The model under review builds one solid part; all positions refer to its coordinate system, in mm. A direction names the side the tool comes from. Round coordinates to 2 decimals unless told otherwise and drop trailing zeros. Order: outer loops, then holes, each group sorted by start corner. A loop starts at its lowest first (then second) coordinate and runs counter-clockwise, first axis right, second up. Notation, with made-up numbers: M 38.25,42.5 L 52.25,42.5 A23 ccw 52.25,60.5 Z; hole C 36.25,65 d10. An arc over 180 degrees is marked long. Use a Markdown table: item, result. Add a question column.
1. Consider section B-B on x = 17. State the section outline as (y, z) points, then the cut area to 3 significant figures.
2. To check wall thickness, follow probe 1 along X at (y, z) = (-95.95, -66); probe 2 along Y at (x, z) = (22, -7); probe 3 along Z at (x, y) = (-8.5, -88). State the ranges of each line that lie inside material, in increasing order.
3. Consider section C-C on z = -43. State the section outline as (x, y) points, then the cut area to 4 significant figures.
4. Consider section D-D on y = -75.5. State the section outline as (x, z) points, then the cut area to 4 significant figures.
5. The part is to be moulded in two halves that separate along X. For faces 6 (the flat face through (15, -96, -70)), 7 (the flat face through (-15.079, -94, -35)), 8 (the flat face through (-3.079, -84, 1)), 9 (the flat face through (38.421, -83, 1)), say which applies: +X half, -X half, draft (parallel to the pull), parting line (faces both ways), or undercut.
6. Insertion check: P1, Ø1.5, axis at x = 19, y = -103, coming from the -Z side; P2, Ø1.7, axis at x = -21.08, y = -115.76, coming from the -Z side; P3, Ø7, axis at y = -92.5, z = -46.5, coming from the -X side; P4, Ø6, axis at x = 6, z = -29, coming from the +Y side. Each pin has a flat end and moves straight along its axis. Give the tip position at first contact, or say it passes through.
7. Consider section A-A on z = -66. State the section outline as (x, y) points.
8. For faces 1 (the flat face through (14, -118.756, 1)), 2 (the flat face through (-13.079, -92, -35)), 3 (the flat face through (27, -76.756, 1)), 4 (the flat face through (53.421, -81, 1)), 5 (the flat face through (44.421, -94, -35)), list the 3-axis set-ups (+Z, -Z, +X, -X, +Y, -Y) from which the entire face can be reached by the end or side of a thin tool; tool diameter is ignored.
from build123d import *

# Parameters (mm, degrees)
SZKIC1_W                    = 77.5
SZKIC1_H                    = 77
SZKIC1_W_2                  = 13.5
SZKIC1_H_2                  = 11
DODANIE_WYCI_GNI_CIE1_DEPTH = 3
DODANIE_WYCI_GNI_CIE3_DEPTH = 70
SZKIC2_R                    = 1.4
WYTNIJ_WYCI_GNI_CIE1_DEPTH  = 3
SZKIC4_R                    = 1.4
WYTNIJ_WYCI_GNI_CIE2_DEPTH  = 3
SZKIC5_R                    = 1.5
WYTNIJ_WYCI_GNI_CIE3_DEPTH  = 5
SFAZOWANIE1_SIZE            = 1
SFAZOWANIE2_SIZE            = 1
SFAZOWANIE3_SIZE            = 1


with BuildPart() as part:
    # Szkic1 → Dodanie-wyciągnięcie1 (new body)
    with BuildSketch(Plane.XY):
        with Locations((14.670842187, -80.255543912)):
            Rectangle(SZKIC1_W, SZKIC1_H)
        with Locations((3.670842187, -84.255543912)):
            Rectangle(SZKIC1_W_2, SZKIC1_H_2, mode=Mode.SUBTRACT)
        Polygon((15.420842187, -76.755543912), (38.420842187, -76.755543912), (38.420842187, -89.755543912), (28.920842187, -89.755543912), (28.920842187, -84.755543912), (15.420842187, -84.755543912), align=None, mode=Mode.SUBTRACT)
    extrude(amount=DODANIE_WYCI_GNI_CIE1_DEPTH)

    # Szkic1<5> → Dodanie-wyciągnięcie3 (add)
    with BuildSketch(Plane.XY):
        Polygon((42.420842187, -89.755543912), (44.420842187, -89.755543912), (44.420842187, -98.755543912), (-15.079157813, -98.755543912), (-15.079157813, -89.755543912), (-13.079157813, -89.755543912), (-13.079157813, -93.755543912), (42.420842187, -93.755543912), align=None)
    extrude(amount=-DODANIE_WYCI_GNI_CIE3_DEPTH)

    # Szkic2 → Wytnij-wyciągnięcie1 (cut)
    with BuildSketch(Plane.XY.offset(3)):
        with Locations((-8.329157813, -44.755543912)):
            Circle(SZKIC2_R)
        with Locations((37.670842187, -44.755543912)):
            Circle(SZKIC2_R)
    extrude(amount=-WYTNIJ_WYCI_GNI_CIE1_DEPTH, mode=Mode.SUBTRACT)

    # Szkic4 → Wytnij-wyciągnięcie2 (cut)
    with BuildSketch(Plane.XY.offset(3)):
        with Locations((-21.079157813, -69.755543912)):
            Circle(SZKIC4_R)
        with Locations((-21.079157813, -115.755543912)):
            Circle(SZKIC4_R)
        with Locations((50.420842187, -115.755543912)):
            Circle(SZKIC4_R)
        with Locations((50.420842187, -69.755543912)):
            Circle(SZKIC4_R)
    extrude(amount=-WYTNIJ_WYCI_GNI_CIE2_DEPTH, mode=Mode.SUBTRACT)

    # Szkic5 → Wytnij-wyciągnięcie3 (cut)
    with BuildSketch(Plane(origin=(0, -93.755543912, 0), x_dir=(1, 0, 0), z_dir=(0, 1, 0))):
        with Locations(Location((34.920842187, 66, 0), (0, 0, 270))):
            Circle(SZKIC5_R)
        with Locations(Location((6.920842187, 66, 0), (0, 0, 270))):
            Circle(SZKIC5_R)
    extrude(amount=-WYTNIJ_WYCI_GNI_CIE3_DEPTH, mode=Mode.SUBTRACT)

    # Sfazowanie1
    sfazowanie1_edges = [part.edges().sort_by_distance(p)[0] for p in [
        (-9.729157813, -44.755543912, 3),
    ]]
    chamfer(sfazowanie1_edges, length=SFAZOWANIE1_SIZE)

    # Sfazowanie2
    sfazowanie2_edges = [part.edges().sort_by_distance(p)[0] for p in [
        (36.270842187, -44.755543912, 3),
    ]]
    chamfer(sfazowanie2_edges, length=SFAZOWANIE2_SIZE)

    # Sfazowanie3
    sfazowanie3_edges = [part.edges().sort_by_distance(p)[0] for p in [
        (49.020842187, -69.755543912, 3),
        (49.020842187, -115.755543912, 3),
        (-22.479157813, -115.755543912, 3),
        (-22.479157813, -69.755543912, 3),
    ]]
    chamfer(sfazowanie3_edges, length=SFAZOWANIE3_SIZE)


solid = part.part
Answer block:
| question | item | result |
|---|---|---|
| 1 | outline | M -118.76,0 L -98.76,0 L -98.76,-70 L -93.76,-70 L -93.76,0 L -84.76,0 L -84.76,3 L -118.76,3 Z; M -76.76,0 L -41.76,0 L -41.76,3 L -76.76,3 Z |
| 1 | area | 557 mm^2 |
| 2 | probe 1 | -15.08 to 5.42, 8.42 to 33.42, 36.42 to 44.42 |
| 2 | probe 2 | -98.76 to -93.76 |
| 2 | probe 3 | 0 to 3 |
| 3 | outline | M -15.08,-98.76 L 44.42,-98.76 L 44.42,-89.76 L 42.42,-89.76 L 42.42,-93.76 L -13.08,-93.76 L -13.08,-89.76 L -15.08,-89.76 Z |
| 3 | area | 313.5 mm^2 |
| 4 | outline | M -24.08,0 L 53.42,0 L 53.42,3 L -24.08,3 Z |
| 4 | area | 232.5 mm^2 |
| 5 | face 6 | draft |
| 5 | face 7 | -X half |
| 5 | face 8 | undercut |
| 5 | face 9 | undercut |
| 6 | P1 | z = 0 |
| 6 | P2 | through |
| 6 | P3 | x = -15.08 |
| 6 | P4 | y = -93.76 |
| 7 | outline | M -15.08,-98.76 L 5.42,-98.76 L 5.42,-93.76 L -13.08,-93.76 L -13.08,-89.76 L -15.08,-89.76 Z; M 8.42,-98.76 L 33.42,-98.76 L 33.42,-93.76 L 8.42,-93.76 Z; M 36.42,-98.76 L 44.42,-98.76 L 44.42,-89.76 L 42.42,-89.76 L 42.42,-93.76 L 36.42,-93.76 Z |
| 8 | face 1 | +Z, -Z, +X, -X, -Y |
| 8 | face 2 | -Z, +Y |
| 8 | face 3 | +Z, -Z |
| 8 | face 4 | +Z, -Z, +X, +Y, -Y |
| 8 | face 5 | -Z, +X, +Y, -Y |
